Geometry check sheet. Reference: drawing and pictorial views, mm from the part's lowest x, y, z. A direction names the side the tool comes from. Give positions to 0.01 mm unless a question says otherwise; leave off trailing zeros. Loops run counter-clockwise (first coordinate to the right, second up) from the corner with the lowest first, then second, coordinate; pieces in that order, holes last. Notation, with made-up numbers: (77, -13.5) -> (120, -13.5) arc R9 ccw to (120, -3.5) -> close; hole circle Ø4 at (5, 82). An arc over 180 degrees is marked (long way). Write item = value, one per line. Start each with the question number.
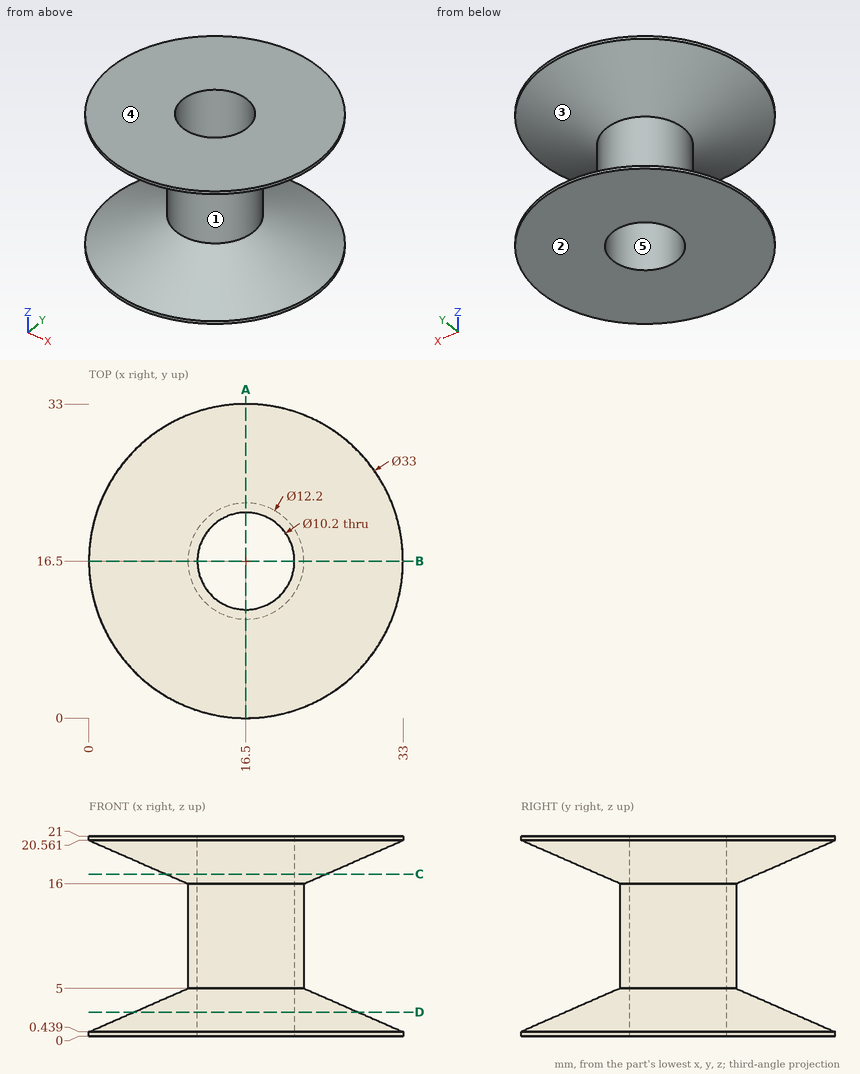
1) Section check D-D (z = 2.5). Enter the section's corners in (x, y).
2) Tool access check on the marked faces 1 and 2. Record the directions out of +Z, -Z, +X, -X, +Y, -Y that give a thin tool (end or side, any length) a straight path to the whole face; none if there is none.
3) Section check A-A (x = 16.5). Enter the section's corners in (y, z).
4) Section check C-C (z = 17). Enter the section's corners in (x, y), plus the area to 3 significant figures.
5) Draft check along X on the marked faces 3, 4 and 5. Enter one of: released by +X, released by -X, zero draft, split by the parting line, or undercut.
6) Thickness scan on line 1 (Y direction, x = 16.5, z = 7); line 2 (Z direction, x = 3.5, y = 22.5) (1 decimal); line 3 (Y direction, x = 16.5, z = 16.75). Record the ranges inside material, lowest first.
Check result:
q1.outline = circle Ø23.6 at (16.5, 16.5); hole circle Ø10.2 at (16.5, 16.5)
q2.face_1 = none
q2.face_2 = -Z, +X, -X, +Y, -Y
q3.outline = (0, 0) -> (11.4, 0) -> (11.4, 21) -> (0, 21) -> (0, 20.56) -> (10.4, 16) -> (10.4, 5) -> (0, 0.44) -> close; (21.6, 0) -> (33, 0) -> (33, 0.44) -> (22.6, 5) -> (22.6, 16) -> (33, 20.56) -> (33, 21) -> (21.6, 21) -> close
q4.outline = circle Ø16.76 at (16.5, 16.5); hole circle Ø10.2 at (16.5, 16.5)
q4.area = 139 mm2
q5.face_3 = split by the parting line
q5.face_4 = zero draft
q5.face_5 = undercut
q6.line_1 = 10.4 to 11.4, 21.6 to 22.6
q6.line_2 = 0 to 1.4, 19.6 to 21
q6.line_3 = 8.69 to 11.4, 21.6 to 24.31
